from build123d import *

# Parameters (mm, degrees)
CROQUIS1_R              = 1.75
SALIENTE_EXTRUIR1_DEPTH = 5
CROQUIS2_R              = 3.493601412
CROQUIS2_W              = 12
CROQUIS2_H              = 6.987202823
SALIENTE_EXTRUIR2_DEPTH = 4.7
CROQUIS3_R              = 1.537305571
CROQUIS3_R_2            = 1.5
SALIENTE_EXTRUIR3_DEPTH = 2


with BuildPart() as part:
    # Croquis1 → Saliente-Extruir1 (new body)
    with BuildSketch(Plane(origin=(0, 0, 0), x_dir=(1, 0, 0), z_dir=(0, 1, 0))):
        with BuildLine():
            Line((36.568555692, 6.987202823), (4.568555692, 6.987202823))
            ThreePointArc((4.568555692, 6.987202823), (1.07495428, 3.493601412), (4.568555692, 0))
            Line((4.568555692, 0), (36.568555692, 0))
            ThreePointArc((36.568555692, 0), (40.062157104, 3.493601412), (36.568555692, 6.987202823))
        make_face()
        with Locations((4.568555692, 3.493601412)):
            Circle(CROQUIS1_R, mode=Mode.SUBTRACT)
        with Locations((36.568555692, 3.493601412)):
            Circle(CROQUIS1_R, mode=Mode.SUBTRACT)
    extrude(amount=SALIENTE_EXTRUIR1_DEPTH)

    # Croquis2 → Saliente-Extruir2 (add)
    with BuildSketch(Plane(origin=(0, 5, 0), x_dir=(1, 0, 0), z_dir=(0, 1, 0))):
        with Locations((26.568555692, 3.493601412)):
            Circle(CROQUIS2_R)
        with Locations((14.568555692, 3.493601412)):
            Circle(CROQUIS2_R)
        with Locations((20.568555692, 3.493601412)):
            Rectangle(CROQUIS2_W, CROQUIS2_H)
    extrude(amount=SALIENTE_EXTRUIR2_DEPTH)

    # Croquis3 → Saliente-Extruir3 (add)
    with BuildSketch(Plane(origin=(0, 9.7, 0), x_dir=(1, 0, 0), z_dir=(0, 1, 0))):
        with BuildLine():
            Line((4.568555692, 6.987202823), (36.568555692, 6.987202823))
            ThreePointArc((36.568555692, 6.987202823), (40.062157104, 3.493601412), (36.568555692, 0))
            Line((36.568555692, 0), (4.568555692, 0))
            ThreePointArc((4.568555692, 0), (1.07495428, 3.493601412), (4.568555692, 6.987202823))
        make_face()
        with Locations((4.568555692, 3.493601412)):
            Circle(CROQUIS3_R, mode=Mode.SUBTRACT)
        with Locations((36.568555692, 3.493601412)):
            Circle(CROQUIS3_R_2, mode=Mode.SUBTRACT)
    extrude(amount=SALIENTE_EXTRUIR3_DEPTH)


solid = part.part
Geometry check sheet. Reference: the model listing, model coordinates, mm. A direction names the side the tool comes from. Give positions to 0.01 mm unless a question says otherwise; leave off trailing zeros. Write each loop counter-clockwise with the first axis right and the second up, starting at its lowest first coordinate (ties: lowest second). Pieces come first, ordered by that corner, then holes. Notation, with made-up numbers: M 13.5,28.5 L 31.5,28.5 A25 ccw 31.5,55.5 Z; hole C 2,56 d3. An arc over 180 degrees is marked long. Answer as CSV lines item,"result". Start each with the question number.
Q1. Tool access check on faces 4 (the face through (4.2, 10.7, -2)), 5 (the face through (34.82, 2.46, -3.57)), 6 (the face through (11.076, 7.317, -3.57)). Record the directions out of +Z, -Z, +X, -X, +Y, -Y that give a thin tool (end or side, any length) a straight path to the whole face; none if there is none.
Q2. Section check C-C, the plane y = 2.5. Record the cut outline in (x, z), then the cut area to 3 significant figures.
Q3. Material ranges on L1, parallel to Y at x = 32.5, z = -0.5; L2, parallel to X at y = 4.25, z = -3.25; L3, parallel to X at y = 0.5, z = -2, recorded low to high.
Q4. Section check B-B, the plane z = -4.5. Record the cut outline in (x, y).
Q5. Go/stop test with flat-tipped pins: pin 1 (2.5 mm diameter, centred on x = 36.57, z = -3.49, fed in from +Y); pin 2 (6 mm diameter, centred on x = 8, y = 6.5, fed in from +Z). Record where each tip stops, or that it passes through.
Q6. Section check D-D, the plane x = 4. Record the cut outline in (y, z), then the cut area to 3 significant figures.
Q7. Release check for a two-part mould opening along Y. For faces 1 (the face through (30.06, 7.32, -3.42)), 2 (the face through (20, 4, -6.987)), 3 (the face through (21, 11.7, -4)) record: pulls with the +Y half, pulls with the -Y half, needs draft (parallel to the pull), parting line crosses it, or undercut.
Q8. Section check A-A, the plane x = 30.5. Record the cut outline in (y, z).
Geometry says:
1,face 4,"+Y, -Y"
1,face 5,"-Y"
1,face 6,"-X"
2,outline,"M 4.57,-6.99 L 36.57,-6.99 A3.49 ccw 36.57,0 L 4.57,0 A3.49 ccw Z; hole C 4.57,-3.49 d3.5; hole C 36.57,-3.49 d3.5"
2,area,"243 mm^2"
3,L1,"0 to 5, 9.7 to 11.7"
3,L2,"1.08 to 2.84, 6.3 to 34.84, 38.3 to 40.05"
3,L3,"1.41 to 3.66, 5.48 to 35.66, 37.48 to 39.73"
4,outline,"M 1.22,0 L 3.14,0 L 3.14,5 L 1.22,5 Z; M 1.22,9.7 L 3.41,9.7 L 3.41,11.7 L 1.22,11.7 Z; M 5.73,9.7 L 11.22,9.7 L 11.22,5 L 6,5 L 6,0 L 35.14,0 L 35.14,5 L 29.91,5 L 29.91,9.7 L 35.46,9.7 L 35.46,11.7 L 5.73,11.7 Z; M 37.68,9.7 L 39.91,9.7 L 39.91,11.7 L 37.68,11.7 Z; M 38,0 L 39.91,0 L 39.91,5 L 38,5 Z"
5,pin 1,"through"
5,pin 2,"z = 0"
6,outline,"M 0,-6.94 L 5,-6.94 L 5,-5.15 L 0,-5.15 Z; M 0,-1.84 L 5,-1.84 L 5,-0.05 L 0,-0.05 Z; M 9.7,-6.94 L 11.7,-6.94 L 11.7,-4.92 L 9.7,-4.92 Z; M 9.7,-2.07 L 11.7,-2.07 L 11.7,-0.05 L 9.7,-0.05 Z"
6,area,"26.0 mm^2"
7,face 1,"undercut"
7,face 2,"needs draft"
7,face 3,"pulls with the +Y half"
8,outline,"M 0,-6.99 L 5,-6.99 L 5,0 L 0,0 Z; M 9.7,-6.99 L 11.7,-6.99 L 11.7,0 L 9.7,0 Z"
